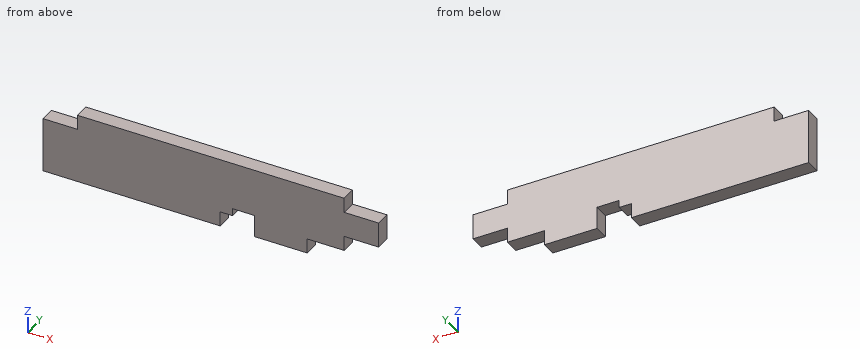
```python
from build123d import *

# Parameters (mm, degrees)
SKETCH1_W           = 863.6
SKETCH1_H           = 179.3875
BOSS_EXTRUDE1_DEPTH = 38.1
SKETCH2_W           = 88.9
SKETCH2_H           = 38.1
CUT_EXTRUDE4_DEPTH  = 39.1
SKETCH3_W           = 184.15
SKETCH3_H           = 38.1
CUT_EXTRUDE1_DEPTH  = 39.1
CUT_EXTRUDE2_DEPTH  = 39.1
SKETCH5_W           = 88.9
SKETCH5_H           = 38.1
CUT_EXTRUDE3_DEPTH  = 39.1
SKETCH6_W           = 88.9
SKETCH6_H           = 38.1
CUT_EXTRUDE5_DEPTH  = 39.1


with BuildPart() as part:
    # Sketch1 → Boss-Extrude1 (new body)
    with BuildSketch(Plane(origin=(0, 0, 0), x_dir=(1, 0, 0), z_dir=(0, 1, 0))):
        with Locations((431.8, 89.69375)):
            Rectangle(SKETCH1_W, SKETCH1_H)
    extrude(amount=BOSS_EXTRUDE1_DEPTH)

    # Sketch2 → Cut-Extrude4 (cut, through all)
    with BuildSketch(Plane.XZ):
        with Locations((819.15, -19.05)):
            Rectangle(SKETCH2_W, SKETCH2_H)
    extrude(amount=-CUT_EXTRUDE4_DEPTH, mode=Mode.SUBTRACT)

    # Sketch3 → Cut-Extrude1 (cut, through all)
    with BuildSketch(Plane.XZ):
        with Locations((771.525, -160.3375)):
            Rectangle(SKETCH3_W, SKETCH3_H)
    extrude(amount=-CUT_EXTRUDE1_DEPTH, mode=Mode.SUBTRACT)

    # Sketch4 → Cut-Extrude2 (cut, through all)
    with BuildSketch(Plane.XZ):
        Polygon((544.56454079, -179.3875), (544.56454079, -122.2375), (487.426, -122.2375), (487.426, -141.2875), (455.676, -141.2875), (455.676, -179.3875), align=None)
    extrude(amount=-CUT_EXTRUDE2_DEPTH, mode=Mode.SUBTRACT)

    # Sketch5 → Cut-Extrude3 (cut, through all)
    with BuildSketch(Plane.XZ):
        with Locations((819.15, -122.2375)):
            Rectangle(SKETCH5_W, SKETCH5_H)
    extrude(amount=-CUT_EXTRUDE3_DEPTH, mode=Mode.SUBTRACT)

    # Sketch6 → Cut-Extrude5 (cut, through all)
    with BuildSketch(Plane(origin=(0, 38.1, 0), x_dir=(1, 0, 0), z_dir=(0, 1, 0))):
        with Locations((44.45, 19.05)):
            Rectangle(SKETCH6_W, SKETCH6_H)
    extrude(amount=-CUT_EXTRUDE5_DEPTH, mode=Mode.SUBTRACT)


solid = part.part
```
Build history of the part. All positions in model axes, mm. Give positions to 0.01 mm unless a question says otherwise; leave off trailing zeros. Loops run counter-clockwise (first coordinate to the right, second up) from the corner with the lowest first, then second, coordinate; pieces in that order, holes last. Notation, with made-up numbers: (30, 48.25) -> (83, 48.25) arc R10 ccw to (83, 54.25) -> close; hole circle Ø11 at (24.5, -22.5). An arc over 180 degrees is marked (long way). One line per question, with ' | ' between items.
Q1. Cut at A-A, the plane y = 30. Write the cut outline in (x, z), plus the area to 3 significant figures.
Filled sheet:
outline: (0, -179.39) -> (455.68, -179.39) -> (455.68, -141.29) -> (487.43, -141.29) -> (487.43, -122.24) -> (544.56, -122.24) -> (544.56, -179.39) -> (679.45, -179.39) -> (679.45, -141.29) -> (774.7, -141.29) -> (774.7, -103.19) -> (863.6, -103.19) -> (863.6, -38.1) -> (774.7, -38.1) -> (774.7, 0) -> (88.9, 0) -> (88.9, -38.1) -> (0, -38.1) -> close | area: 133,000 mm²
Q2. Cut at C-C, the plane x = 497. Write the cut outline in (y, z), plus the area to 3 significant figures.
Filled sheet:
outline: (0, -122.24) -> (38.1, -122.24) -> (38.1, 0) -> (0, 0) -> close | area: 4,660 mm²
Q3. Drop flat-ended pins along their axis: pin 1 (19 mm diameter, centred on x = 829, y = 12.5, fed in from +Z); pin 2 (19 mm diameter, centred on y = 14.5, z = -169.5, fed in from +X); pin 3 (3 mm diameter, centred on y = 15.5, z = -27.5, fed in from -X). Give the stop position or say it passes through.
Filled sheet:
pin 1: stops at z = -38.1 | pin 2: stops at x = 679.45 | pin 3: stops at x = 88.9
Q4. Cut at B-B, the plane x = 740.5. Write the cut outline in (y, z).
Filled sheet:
outline: (0, -141.29) -> (38.1, -141.29) -> (38.1, 0) -> (0, 0) -> close
Q5. Drill centre lines: line 1 along X through (y, z) = (36, -155); line 2 along Z through (x, y) = (58, 32); line 3 along Z through (x, y) = (510.5, 32). Where is each one in solid material? Low to high. Write a range as [from, to].
Filled sheet:
line 1: x = [0, 455.68], [544.56, 679.45] | line 2: z = [-179.39, -38.1] | line 3: z = [-122.24, 0]
